Study the drawing (mm; zero at the part's minimum x, y, z) and answer. Give positions to 0.01 mm unless a question says otherwise; leave off trailing zeros. Loops run counter-clockwise (first coordinate to the right, second up) from the corner with the lowest first, then second, coordinate; pieces in that order, holes last. Notation, with made-up numbers: (42, -17.5) - (62, -17.5) arc R31 cw to (62, 7.5) - close; hole circle Ø4 at (-29.5, 41.25). An arc over 180 degrees is marked (long way). Write item = value, one per line. Start each with the question number.
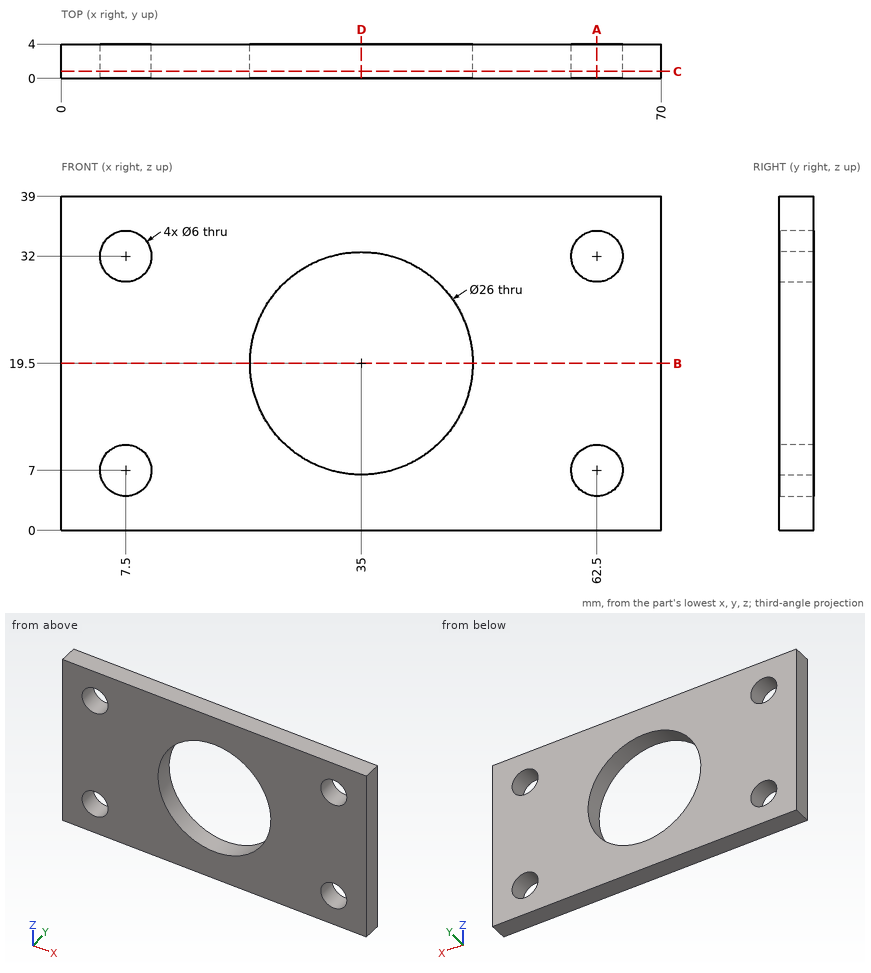
1. Consider line 1 along X through (y, z) = (2.8, 19.5); line 2 along X through (y, z) = (1.05, 31.5); line 3 along Z through (x, y) = (5.5, 2.25). Determine where each line is inside the solid, lowest interval first. Write a range as [from, to].
2. A cutting plane is placed at C-C on y = 0.8. Give the vertices of the cut face in (x, z).
3. A cutting plane is placed at D-D on x = 35. Give the vertices of the cut face in (y, z), and give its area (3 significant figures).
4. A cutting plane is placed at B-B on z = 19.5. Give the vertices of the cut face in (x, y).
5. A cutting plane is placed at A-A on x = 62.5. Give the vertices of the cut face in (y, z).
6. Given P1, Ø6, axis at x = 15.5, z = 23.5, coming from the -Y side, flat-ended and moving along its own axis, determine where the tip first touches the part or whether it passes through.
Reply:
q1.line_1 = [0, 22], [48, 70]
q1.line_2 = [0, 4.54], [10.46, 30], [40, 59.54], [65.46, 70]
q1.line_3 = [0, 4.76], [9.24, 29.76], [34.24, 39]
q2.outline = (0, 0) - (70, 0) - (70, 39) - (0, 39) - close; hole circle Ø6 at (7.5, 7); hole circle Ø6 at (7.5, 32); hole circle Ø26 at (35, 19.5); hole circle Ø6 at (62.5, 7); hole circle Ø6 at (62.5, 32)
q3.outline = (0, 0) - (4, 0) - (4, 6.5) - (0, 6.5) - close; (0, 32.5) - (4, 32.5) - (4, 39) - (0, 39) - close
q3.area = 52.0 mm^2
q4.outline = (0, 0) - (22, 0) - (22, 4) - (0, 4) - close; (48, 0) - (70, 0) - (70, 4) - (48, 4) - close
q5.outline = (0, 0) - (4, 0) - (4, 4) - (0, 4) - close; (0, 10) - (4, 10) - (4, 29) - (0, 29) - close; (0, 35) - (4, 35) - (4, 39) - (0, 39) - close
q6.P1 = 0
